from build123d import *

# Parameters (mm, degrees)
SKETCH1_R                       = 50
BOSS_EXTRUDE1_DEPTH             = 2
BOSS_EXTRUDE3_START             = -2
BOSS_EXTRUDE3_DEPTH             = 2
SKETCH4_R                       = 4.5
SKETCH4_R_2                     = 2.55
BOSS_EXTRUDE2_DEPTH             = 10
CIRPATTERN2_COUNT               = 4
CIRPATTERN2_ANGLE               = 180
CUT_EXTRUDE2_REACH              = 75.186
CIRPATTERN3_COUNT               = 3
CIRPATTERN3_ANGLE               = 120
CIRPATTERN3_THE_OTHER_WAY_COUNT = 3
CIRPATTERN3_THE_OTHER_WAY_ANGLE = 120
FILLET1_R                       = 10
FILLET2_R                       = 1


with BuildPart() as part:
    # Sketch1 → Boss-Extrude1 (new body)
    with BuildSketch(Plane.XY):
        Circle(SKETCH1_R)
    extrude(amount=BOSS_EXTRUDE1_DEPTH)

    # Sketch5 → Boss-Extrude3 (add)
    with BuildSketch(Plane.XY.offset(2).offset(BOSS_EXTRUDE3_START)):
        with BuildLine():
            Line((-2.847377425, 49.918858579), (-3, 52.414215629))
            ThreePointArc((-3, 52.414215629), (0, 52.5), (3, 52.414215629))
            Line((3, 52.414215629), (2.847377425, 49.918858579))
            ThreePointArc((2.847377425, 49.918858579), (0, 50), (-2.847377425, 49.918858579))
        make_face()
    boss_extrude3 = extrude(amount=BOSS_EXTRUDE3_DEPTH)

    # Sketch4 → Boss-Extrude2 (add)
    with BuildSketch(Plane.XY.offset(2)):
        Circle(SKETCH4_R)
        Circle(SKETCH4_R_2, mode=Mode.SUBTRACT)
    extrude(amount=BOSS_EXTRUDE2_DEPTH)

    # CirPattern2: Boss-Extrude3 ×4 about axis
    cirpattern2_axis = Axis((0, 0, 0), (0, 0, -1))
    for i in range(1, CIRPATTERN2_COUNT):
        add(boss_extrude3.rotate(cirpattern2_axis, i * CIRPATTERN2_ANGLE / (CIRPATTERN2_COUNT - 1)))

    # Sketch7 → Cut-Extrude2 (cut, up to next)
    with BuildSketch(Plane.XY.offset(2), mode=Mode.PRIVATE) as cut_extrude2_sk1:
        with BuildLine():
            Line((48.293213683, 12.952432674), (25.188266684, 6.761480784))
            ThreePointArc((25.188266684, 6.761480784), (20, 0), (25.188266684, -6.761480784))
            Line((25.188266684, -6.761480784), (48.293213683, -12.952432674))
            ThreePointArc((48.293213683, -12.952432674), (50, 0), (48.293213683, 12.952432674))
        make_face()
    cut_extrude2_tool1 = extrude(cut_extrude2_sk1.sketch, amount=-CUT_EXTRUDE2_REACH, mode=Mode.PRIVATE) & part.part
    cut_extrude2 = cut_extrude2_tool1.solids().sort_by_distance((37.115477, 0, 2))[0]
    add(cut_extrude2, mode=Mode.SUBTRACT)

    # CirPattern3: Cut-Extrude2 ×3 about axis
    cirpattern3_axis = Axis((0, 0, 0), (0, 0, 1))
    for i in range(1, CIRPATTERN3_COUNT):
        add(cut_extrude2.rotate(cirpattern3_axis, i * CIRPATTERN3_ANGLE / (CIRPATTERN3_COUNT - 1)), mode=Mode.SUBTRACT)

    # CirPattern3 the other way: Cut-Extrude2 ×3 about axis
    cirpattern3_the_other_way_axis = Axis((0, 0, 0), (0, 0, -1))
    for i in range(1, CIRPATTERN3_THE_OTHER_WAY_COUNT):
        add(cut_extrude2.rotate(cirpattern3_the_other_way_axis, i * CIRPATTERN3_THE_OTHER_WAY_ANGLE / (CIRPATTERN3_THE_OTHER_WAY_COUNT - 1)), mode=Mode.SUBTRACT)

    # Fillet1
    # the kernel refuses this fillet: 10 mm, written as the material it takes off along each edge
    with BuildSketch(Plane(origin=(-35.363742578, 35.346933543, 33.509652434), x_dir=(-0.6121571340688006, -0.7907361400673886, 0), z_dir=(0, 0, -1))) as fillet1_piece_1:
        with BuildLine():
            CenterArc((11.343474876, -9.920253368), FILLET1_R, 82.759261871, 104.49509636)
            Line((1.423521402, -11.182997629), (1.225122333, -11.208252514))
            Line((1.225122333, -11.208252514), (-0.198399069, -0.025254885))
            Line((-0.198399069, -0.025254885), (-0.025207722, 0.198405067))
            ThreePointArc((-0.025207722, 0.198405067), (6.301930487, 0.59873316), (12.629068696, 0.198405067))
            Line((12.629068696, 0.198405067), (12.603860974, 0))
        make_face()
    extrude(amount=65.019304869, mode=Mode.SUBTRACT)
    with BuildSketch(Plane(origin=(-12.929471105, 48.299366217, 29.609711649), x_dir=(0.9873433189599674, 0.15859751103064706, 0), z_dir=(0, 0, -1))) as fillet1_piece_2:
        with BuildLine():
            CenterArc((11.077824317, 9.96238911), FILLET1_R, 174.125500121, 90.903649981)
            Line((1.130339641, 10.985887341), (0.931389948, 11.006357306))
            Line((0.931389948, 11.006357306), (-0.198949694, 0.020469965))
            Line((-0.198949694, 0.020469965), (-0.020422671, -0.198954554))
            ThreePointArc((-0.020422671, -0.198954554), (5.105667647, -0.46136152), (10.194005514, -0.199247782))
            Line((10.194005514, -0.199247782), (10.211335295, 0))
        make_face()
    extrude(amount=57.219423297, mode=Mode.SUBTRACT)
    with BuildSketch(Plane(origin=(35.363742578, -35.346933543, 29.609711649), x_dir=(0.6310211330095078, 0.775765640960849, 0), z_dir=(0, 0, -1)), Plane(origin=(-12.929471105, -48.299366217, 29.609711649), x_dir=(0.9873433189599667, -0.1585975110306507, 0), z_dir=(0, 0, -1)), Plane(origin=(12.929471105, 48.299366217, 29.609711649), x_dir=(-0.987343318959968, 0.15859751103064254, 0), z_dir=(0, 0, -1)), Plane(origin=(48.293213683, 12.952432674, 29.609711649), x_dir=(-0.35632218595046244, 0.9343631519914962, 0), z_dir=(0, 0, -1))) as fillet1_piece_3:
        with BuildLine():
            CenterArc((11.077824317, -9.96238911), FILLET1_R, 94.970849897, 90.903649981)
            Line((1.130339641, -10.985887341), (0.931389948, -11.006357306))
            Line((0.931389948, -11.006357306), (-0.198949694, -0.020469965))
            Line((-0.198949694, -0.020469965), (-0.020422671, 0.198954554))
            ThreePointArc((-0.020422671, 0.198954554), (5.105667647, 0.46136152), (10.194005514, 0.199247782))
            Line((10.194005514, 0.199247782), (10.211335295, 0))
        make_face()
    extrude(amount=57.219423297, mode=Mode.SUBTRACT)
    with BuildSketch(Plane(origin=(12.929471105, -48.299366217, 29.609711649), x_dir=(-0.2588190451025242, 0.9659258262890674, 0), z_dir=(0, 0, -1)), Plane(origin=(35.363742578, 35.346933543, 29.609711649), x_dir=(-0.7071067811865411, -0.707106781186554, 0), z_dir=(0, 0, -1)), Plane(origin=(48.293213683, -12.952432674, 29.609711649), x_dir=(-0.96592582628907, 0.2588190451025145, 0), z_dir=(0, 0, -1))) as fillet1_piece_4:
        with BuildLine():
            CenterArc((11.043884659, -10), FILLET1_R, 90, 90.903649981)
            Line((1.045128361, -10.157710136), (0.845153235, -10.160864339))
            ThreePointArc((0.845153235, -10.160864339), (0.063625516, -5.126075338), (-0.199999994, -4.7543e-05))
            Line((-0.199999994, -4.7543e-05), (0, 0.2))
            Line((0, 0.2), (11.043884659, 0.2))
            Line((11.043884659, 0.2), (11.043884659, 0))
        make_face()
    extrude(amount=57.219423297, mode=Mode.SUBTRACT)
    with BuildSketch(Plane(origin=(-35.363742578, -35.346933543, 33.509652434), x_dir=(0.7071067811865469, 0.7071067811865481, 0), z_dir=(0, 0, -1))) as fillet1_piece_5:
        with BuildLine():
            CenterArc((11.273235967, -10), FILLET1_R, 90, 104.49509636)
            Line((1.591545311, -12.502971446), (1.397911498, -12.553030874))
            ThreePointArc((1.397911498, -12.553030874), (0.201832147, -6.327090409), (-0.199999994, -4.7543e-05))
            Line((-0.199999994, -4.7543e-05), (0, 0.2))
            Line((0, 0.2), (11.273235967, 0.2))
            Line((11.273235967, 0.2), (11.273235967, 0))
        make_face()
    extrude(amount=65.019304869, mode=Mode.SUBTRACT)

    # Fillet2
    fillet2_edges = [part.edges().sort_by_distance(p)[0] for p in [
        (-2.55, 0, 2),
        (-4.5, 0, 2),
    ]]
    fillet(fillet2_edges, radius=FILLET2_R)


solid = part.part
Design review of the part built by this model. Coordinates are the model's own, in mm. A direction names the side the tool comes from. Coordinates: 2 decimals unless noted, no trailing zeros. Write each loop counter-clockwise with the first axis right and the second up, starting at its lowest first coordinate (ties: lowest second). Pieces come first, ordered by that corner, then holes. Notation, with made-up numbers: (26, 46.25) - (68, 46.25) arc R19 cw to (68, 54.25) - close; hole circle Ø10 at (29, -8.75). An arc over 180 degrees is marked (long way). Use one line per item in the form item = value.
Q1. Insertion check: pin 1 Ø6.5 at (x, y) = (0, 0) entering from -Z; pin 2 Ø3 at (x, y) = (31, 15.5) entering from +Z; pin 3 Ø2 at (x, y) = (-0.5, 1) entering from +Z. Each pin has a flat end and moves straight along its axis. Give the tip position at first contact, or say it passes through.
Taken from the geometry:
pin_1 = 0
pin_2 = 2
pin_3 = 2.18
Q2. Consider section B-B (z = 10.75). Write out the cut boundary in (x, y), plus the area to 3 significant figures.
Taken from the geometry:
outline = circle Ø9 at (0, 0); hole circle Ø5.1 at (0, 0)
area = 43.2 mm^2
Q3. Machinability: for faces 1 (the flat face through (-22.984, 22.967, 1.014)), 2 (the cylindrical face through (1.18, -2.26, 7.44)), 3 (the flat face through (-8.43, -31.5, 1.01)), 4 (the flat face through (31.49, 8.45, 1.01)), which of the approach directions +Z, -Z, +X, -X, +Y, -Y give a long, thin tool a straight path to every point of the face, cutting with its end or side? Answer none if there is none.
Taken from the geometry:
face_1 = +Z, -Z, +Y
face_2 = +Z
face_3 = +Z, -Z
face_4 = +Z, -Z, +X
Q4. Consider section A-A (y = 0). Write out the cut boundary in (x, z).
Taken from the geometry:
outline = (-50, 0) - (20, 0) - (20, 2) - (5.5, 2) arc R1 cw to (4.5, 3) - (4.5, 12) - (2.55, 12) - (2.55, 3) arc R1 cw to (1.55, 2) - (-1.55, 2) arc R1 cw to (-2.55, 3) - (-2.55, 12) - (-4.5, 12) - (-4.5, 3) arc R1 cw to (-5.5, 2) - (-50, 2) - close
Q5. Consider section C-C (x = 40.5). Write out the cut boundary in (y, z).
Taken from the geometry:
outline = (-28.56, 0) - (-11.38, 0) - (-11.38, 2) - (-28.56, 2) - close; (11.38, 0) - (28.56, 0) - (28.56, 2) - (11.38, 2) - close
Q6. Consider section D-D (x = 0). Write out the cut boundary in (y, z), plus the area to 3 significant figures.
Taken from the geometry:
outline = (-52.5, 0) - (52.5, 0) - (52.5, 2) - (5.5, 2) arc R1 cw to (4.5, 3) - (4.5, 12) - (2.55, 12) - (2.55, 3) arc R1 cw to (1.55, 2) - (-1.55, 2) arc R1 cw to (-2.55, 3) - (-2.55, 12) - (-4.5, 12) - (-4.5, 3) arc R1 cw to (-5.5, 2) - (-52.5, 2) - close
area = 250 mm^2
Q7. For probe 1 along Y at (x, z) = (0, 7); probe 2 along Z at (x, y) = (-2.5, -14); probe 3 along X at (y, z) = (18.5, 1.5), list the stretches that pass through material, from the lowest coordinate up.
Taken from the geometry:
probe_1 = -4.5 to -2.55, 2.55 to 4.5
probe_2 = 0 to 2
probe_3 = -46.45 to -18.52, -8.48 to 8.48, 18.52 to 44.96
Q8. The part is to be moulded in two halves that separate along Y. For faces 5 (the cylindrical face through (-50, 0, 1)), 6 (the flat face through (8.43, 31.5, 1.01)), 7 (the cylindrical face through (45.49, -26.21, 0.99)), say which applies: +Y half, -Y half, draft (parallel to the pull), parting line (faces both ways), or undercut.
Taken from the geometry:
face_5 = parting line
face_6 = undercut
face_7 = -Y half
